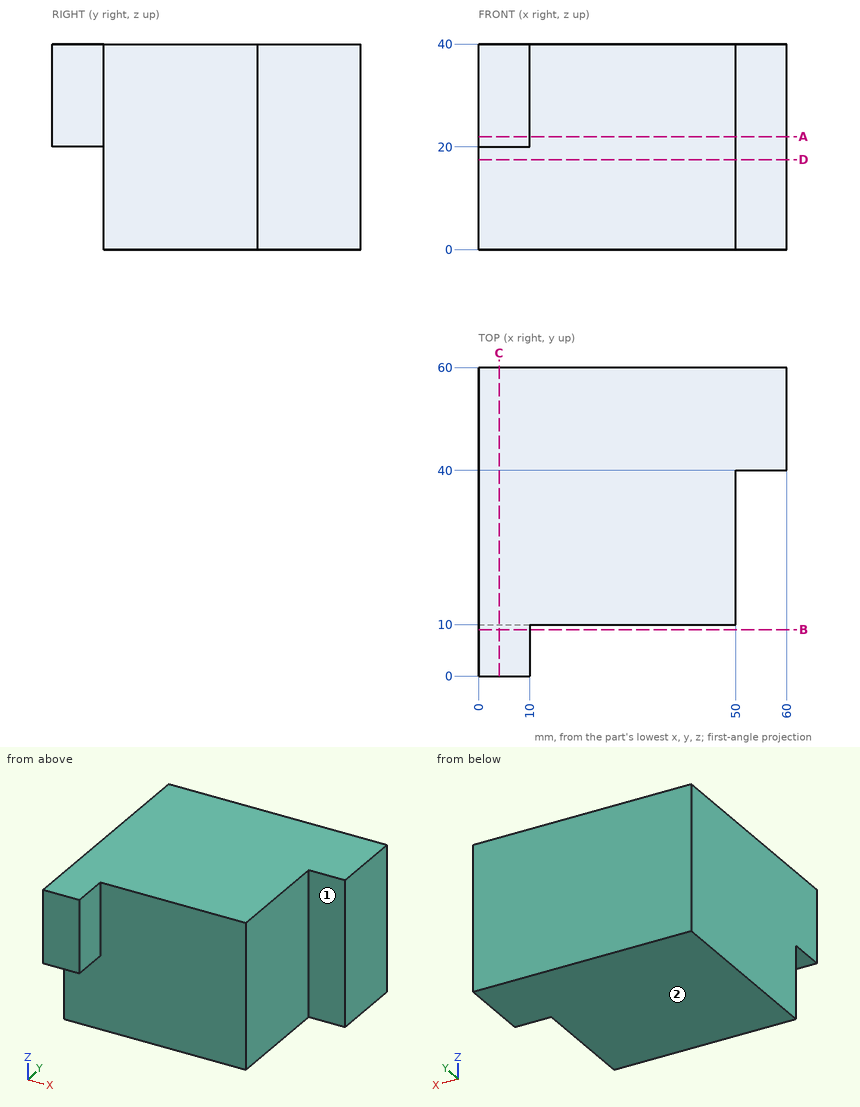
Study the drawing (mm; zero at the part's minimum x, y, z) and answer. A direction names the side the tool comes from. Coordinates: 2 decimals unless noted, no trailing zeros. Loops run counter-clockwise (first coordinate to the right, second up) from the corner with the lowest first, then second, coordinate; pieces in that order, holes last. Notation, with made-up numbers: M 40.5,56.25 L 72.5,56.25 A35 cw 72.5,92.25 Z; hole C 12,53.5 d4. An arc over 180 degrees is marked long. Answer in a Markdown table with one row per item.
1) Find section B-B (y = 9). Determine the outline of the cut face in (x, z), then the cut area to 3 significant figures.
Answers below:
| item | result |
|---|---|
| outline | M 0,20 L 10,20 L 10,40 L 0,40 Z |
| area | 200 mm^2 |
2) Find section D-D (z = 17.5). Determine the outline of the cut face in (x, y), then the cut area to 3 significant figures.
Answers below:
| item | result |
|---|---|
| outline | M 0,10 L 50,10 L 50,40 L 60,40 L 60,60 L 0,60 Z |
| area | 2,700 mm^2 |
3) Which of the six approach directions +Z, -Z, +X, -X, +Y, -Y give full straight-line access (tool end or side, diameter ignored) to the marked faces 1 and 2?
Answers below:
| item | result |
|---|---|
| face 1 | +Z, -Z, +X, -Y |
| face 2 | -Z, +X, -X, +Y, -Y |
4) Find section C-C (x = 4). Determine the outline of the cut face in (y, z), then the cut area to 3 significant figures.
Answers below:
| item | result |
|---|---|
| outline | M 0,20 L 10,20 L 10,0 L 60,0 L 60,40 L 0,40 Z |
| area | 2,200 mm^2 |
5) Given pin 1 (1.5 mm diameter, centred on y = 10, z = 12.5, fed in from +X); pin 2 (1.5 mm diameter, centred on x = 23, y = 37.5, fed in from -Z); pin 3 (5 mm diameter, centred on y = 6.5, z = 27, fed in from +X); pin 4 (5 mm diameter, centred on x = 4, y = 2.5, fed in from -Z), each flat-ended and moving along its own axis, determine where each tip first touches the part or whether it passes through.
Answers below:
| item | result |
|---|---|
| pin 1 | x = 50 |
| pin 2 | z = 0 |
| pin 3 | x = 10 |
| pin 4 | z = 20 |
6) Find section A-A (z = 22). Determine the outline of the cut face in (x, y), then the cut area to 3 significant figures.
Answers below:
| item | result |
|---|---|
| outline | M 0,0 L 10,0 L 10,10 L 50,10 L 50,40 L 60,40 L 60,60 L 0,60 Z |
| area | 2,800 mm^2 |
7) Find the intervals of material crossed by probe 1 along Y at (x, z) = (14.5, 3); probe 2 along X at (y, z) = (6, 26); probe 3 along X at (y, z) = (21, 30), in increasing order.
Answers below:
| item | result |
|---|---|
| probe 1 | 10 to 60 |
| probe 2 | 0 to 10 |
| probe 3 | 0 to 50 |
